The listing builds one solid part. Answer for the finished solid, in the listing's coordinates (mm). A direction names the side the tool comes from. Coordinates: 2 decimals unless noted, no trailing zeros. Write each loop counter-clockwise with the first axis right and the second up, starting at its lowest first coordinate (ties: lowest second). Pieces come first, ordered by that corner, then holes.
(1) The part is cut by section D-D on y = 0. Determine the outline of the cut face in (x, z), plus the area to 3 significant figures.
(2) The part is cut by section A-A on x = 3. Determine the outline of the cut face in (y, z).
(3) The part is cut by section B-B on y = 2.5. Determine the outline of the cut face in (x, z), plus the area to 3 significant figures.
(4) Which of the six approach directions +Z, -Z, +X, -X, +Y, -Y give full straight-line access (tool end or side, diameter ignored) to faces 1 (the flat face through (3, 2, -16.924)), 2 (the flat face through (3, -2.028, -11)), 3 (the cylindrical face through (2, -0.37, 8.65))?
(5) For a pull along X with two mould halves and no side action, classify faces 4 (the flat face through (3, 1.372, -12)), 5 (the cylindrical face through (1.947, -2.916, -14.374)), 6 (the flat face through (6, 0, -2)) as +X half, -X half, draft (parallel to the pull), parting line (faces both ways), or undercut.
(6) Given P1, Ø1.7, axis at x = 3, z = -14.33, coming from the -Y side; P2, Ø1, axis at x = 2, y = 0, coming from the -Z side, each flat-ended and moving along its own axis, determine where each tip first touches the part or whether it passes through.
(7) The part is cut by section C-C on x = 5.45. Determine the outline of the cut face in (y, z), plus the area to 3 significant figures.
(8) Straight lines are drawn through the part: line 1 (Y direction, x = 5.2, z = -7.5); line 2 (Z direction, x = 3, y = 2.7); line 3 (Z direction, x = 3.5, y = -0.25). For each, find the intervals that lie inside material, in ascending order.
Autodesk Inventor part; units mm, degrees
ref_plane "YZ Plane" through (0, 0, 0) normal (1, 0, 0) x (0, 1, 0)
ref_plane "XZ Plane" through (0, 0, 0) normal (0, 1, 0) x (-1, 0, 0)
ref_plane "XY Plane" through (0, 0, 0) normal (0, 0, 1) x (1, 0, 0)
sketch "Sketch1" plane through (0, 0, 0) normal (1, 0, 0) x (0, 1, 0)
  point P0 (0, 0)
sketch "Sketch2" plane through (0, 0, 0) normal (1, 0, 0) x (0, 1, 0)
  line L0 (3.1716, 6.9287) -> (-3.8284, 6.9287)
  line L1 (3.1716, 6.9287) -> (3.1716, -16.9242)
  line L2 (3.1716, -16.9242) -> (1.3716, -16.9242)
  line L3 (1.3716, -16.9242) -> (1.3716, -5.9694)
  line L4 (1.3716, -5.9694) -> (-2.0284, -5.9694)
  line L5 (-2.0284, -5.9694) -> (-2.0284, -16.9242)
  line L6 (-2.0284, -16.9242) -> (-3.8284, -16.9242)
  line L7 (-3.8284, -16.9242) -> (-3.8284, 6.9287)
  point P0 (0, 0)
  dimension "d0" = 7
  dimension "d2" = 1.8
  dimension "d6" = 3.4
  dimension "d8" = 1.8
extrude "Extrusion1" add sketch "Sketch2" along normal blind 6
sketch "Sketch3" plane through (0, 3.1716, 6.9287) normal (0, 1, 0) x (1, 0, 0)
  line L0 (0, 23.8529) -> (6, 23.8529)
  circle A0 centre (3, 32.5) radius 1
  point P0 (0, 6.9287)
  dimension "d12" = 2
extrude "Extrusion2" cut sketch "Sketch3" against normal blind 9.875
sketch "Sketch5" plane through (0, 3.1716, 6.9287) normal (0, 1, 0) x (1, 0, 0)
  point P0 (0, 6.9287)
sketch "Sketch7" plane through (0, -3.8284, 6.9287) normal (0, 0, 1) x (1, 0, 0)
  line L0 (0, 1.8) -> (0, 5.2)
  line L1 (0, 3.5) -> (6, 3.5)
  line L2 (6, 1.8) -> (6, 5.2)
  line L3 (0, 0) -> (6, 0)
  line L4 (3, 0) -> (3, 7)
  line L5 (2, 7) -> (4, 7)
  circle A0 centre (3, 3.5) radius 1
  point P0 (0, 3.8284)
  dimension "d21" = 2
extrude "Extrusion5" add sketch "Sketch7" along normal blind 3.5
sketch "Sketch8" plane through (0, 3.1716, 6.9287) normal (0, 1, 0) x (1, 0, 0)
  line L0 (0, 0) -> (0, 23.8529)
  line L1 (0, 21.256) -> (5.958, 21.256)
  line L2 (5.958, 21.256) -> (3, 23.8529)
  line L3 (0, 23.8529) -> (6, 23.8529)
  line L4 (3, 23.8529) -> (3, 17.8866)
  circle A0 centre (3, 21.256) radius 1.0543
  point P0 (0, 6.9287)
extrude "Extrusion6" cut sketch "Sketch8" against normal blind 39.2125 contours A0 L4 L1 | L1 L4 A0 | L4 A0 L1 | L1 A0 L4
properties part number "Link2"
Model answer:
1. outline: (0, -5.97) - (6, -5.97) - (6, 6.93) - (3.94, 6.93) - (3.94, 10.43) - (2.06, 10.43) - (2.06, 6.93) - (0, 6.93) - close
1. area: 84.0 mm2
2. outline: (-3.83, -16.92) - (-2.03, -16.92) - (-2.03, -15.38) - (-3.83, -15.38) - close; (-3.83, -13.27) - (-2.03, -13.27) - (-2.03, -5.97) - (1.37, -5.97) - (1.37, -13.27) - (3.17, -13.27) - (3.17, 6.93) - (0.67, 6.93) - (0.67, 10.43) - (-1.33, 10.43) - (-1.33, 6.93) - (-3.83, 6.93) - close; (1.37, -16.92) - (3.17, -16.92) - (3.17, -15.38) - (1.37, -15.38) - close
3. outline: (0, -16.92) - (6, -16.92) - (6, 6.93) - (0, 6.93) - close; hole circle Ø2.11 at (3, -14.33)
3. area: 140 mm2
4. face 1: -Z, +X, -X, +Y, -Y
4. face 2: -Z, +X, -X
4. face 3: +Z
5. face 4: draft
5. face 5: undercut
5. face 6: +X half
6. P1: passes through
6. P2: stops at z = -5.97
7. outline: (-3.83, -16.92) - (-2.03, -16.92) - (-2.03, -5.97) - (1.37, -5.97) - (1.37, -16.92) - (3.17, -16.92) - (3.17, 6.93) - (-3.83, 6.93) - close
7. area: 130 mm2
8. line 1: y = -3.83 to -2.03, 1.37 to 3.17
8. line 2: z = -16.92 to -15.38, -13.27 to 6.93
8. line 3: z = -5.97 to 10.43
